The listing builds one solid part. Answer for the finished solid, in the listing's coordinates (mm). A direction names the side the tool comes from. Round coordinates to 2 decimals unless told otherwise and drop trailing zeros. Order: outer loops, then holes, each group sorted by start corner. A loop starts at its lowest first (then second) coordinate and runs counter-clockwise, first axis right, second up. Notation, with made-up numbers: (23.5, 75) - (67.5, 75) arc R19 cw to (67.5, 99) - close; hole circle Ø1 at (24.5, -30). An arc over 180 degrees is marked (long way). Write item = value, one per line.
from build123d import *

# Parameters (mm, degrees)
ESBO_O1_R                     = 35
ESBO_O1_R_2                   = 32.5
RESSALTO_EXTRUS_O1_DEPTH      = 8
RESSALTO_EXTRUS_O2_START      = -3
ESBO_O2_R                     = 32.5
RESSALTO_EXTRUS_O2_DEPTH      = 3
ESBO_O3_R                     = 2.5
CORTE_EXTRUS_O1_DEPTH         = 3
RESSALTO_EXTRUS_O3_DEPTH      = 5
RESSALTO_EXTRUS_O3_DEPTH_BACK = 3
ESBO_O4_R                     = 37
ESBO_O4_R_2                   = 35
ESBO_O5_W                     = 1.8
ESBO_O5_H                     = 3
ESBO_O6_R                     = 12.55
RESSALTO_EXTRUS_O4_DEPTH      = 5
CORTE_EXTRUS_O2_DEPTH         = 53.933921071
CORTE_EXTRUS_O2_DEPTH_BACK    = 53.933921071
ESBO_O7_R                     = 7.55
RESSALTO_EXTRUS_O5_START      = -8
ESBO_O8_R                     = 37
ESBO_O8_R_2                   = 32.5
RESSALTO_EXTRUS_O5_DEPTH      = 8
ESBO_O9_R                     = 37
ESBO_O9_R_2                   = 33.5
CORTE_EXTRUS_O8_DEPTH         = 1.5
CORTE_EXTRUS_O9_START         = -1.5
ESBO_O12_R                    = 37
ESBO_O12_R_2                  = 33.5
CORTE_EXTRUS_O9_DEPTH         = 1.5
CORTE_EXTRUS_O10_START        = -10
ESBO_O13_R                    = 37
ESBO_O13_R_2                  = 36
CORTE_EXTRUS_O10_DEPTH        = 10
ESBO_O14_R                    = 37
ESBO_O14_R_2                  = 36
RESSALTO_EXTRUS_O6_DEPTH      = 5
ESBO_O15_R                    = 12.55
CORTE_EXTRUS_O11_DEPTH        = 53.933921071
ESBO_O16_R                    = 12.55
RESSALTO_EXTRUS_O7_DEPTH      = 3
ESBO_O17_R                    = 10
RESSALTO_EXTRUS_O8_DEPTH      = 16
ESBO_O18_R                    = 2.5
CORTE_EXTRUS_O12_DEPTH        = 56.668662639
ESBO_O19_W                    = 5.95
ESBO_O19_H                    = 2.65
CORTE_EXTRUS_O13_DEPTH        = 8
CORTE_EXTRUS_O14_DEPTH        = 57.676714795
CORTE_EXTRUS_O14_DEPTH_BACK   = 57.676714795
ESBO_O21_R                    = 1.65
ESBO_O23_R                    = 37
ESBO_O23_R_2                  = 36
CORTE_EXTRUS_O15_DEPTH        = 54.798234195


with BuildPart() as part:
    # Esboço1 → Ressalto-extrusão1 (new body)
    with BuildSketch(Plane.XY):
        Circle(ESBO_O1_R)
        Circle(ESBO_O1_R_2, mode=Mode.SUBTRACT)
    extrude(amount=RESSALTO_EXTRUS_O1_DEPTH)

    # Esboço2 → Ressalto-extrusão2 (add)
    with BuildSketch(Plane.XY.offset(8).offset(RESSALTO_EXTRUS_O2_START)):
        Circle(ESBO_O2_R)
    extrude(amount=RESSALTO_EXTRUS_O2_DEPTH)

    # Esboço3 → Corte-extrusão1 (cut)
    with BuildSketch(Plane.XY.offset(8)):
        Circle(ESBO_O3_R)
    extrude(amount=-CORTE_EXTRUS_O1_DEPTH, mode=Mode.SUBTRACT)

    # Esboço4 → Ressalto-extrusão3 (add, two sides: drawn at the far end of the back side and taken through both)
    with BuildSketch(Plane(origin=(0, 0, 5), x_dir=(-1, 0, 0), z_dir=(0, 0, -1)).offset(-RESSALTO_EXTRUS_O3_DEPTH_BACK)):
        Circle(ESBO_O4_R)
        Circle(ESBO_O4_R_2, mode=Mode.SUBTRACT)
    extrude(amount=RESSALTO_EXTRUS_O3_DEPTH + RESSALTO_EXTRUS_O3_DEPTH_BACK)

    # Esboço5 → Corte-Revolução1 (revolve, cut)
    with BuildSketch(Plane(origin=(0, 0, 0), x_dir=(1, 0, 0), z_dir=(0, 1, 0))):
        with Locations((-36.1, -2.5)):
            Rectangle(ESBO_O5_W, ESBO_O5_H)
        with Locations((-36.1, -5.5)):
            Rectangle(ESBO_O5_W, ESBO_O5_H)
    revolve(axis=Axis((0, 0, 8), (0, 0, -1)), mode=Mode.SUBTRACT)

    # Esboço6 → Ressalto-extrusão4 (add)
    with BuildSketch(Plane(origin=(0, 0, 5), x_dir=(-1, 0, 0), z_dir=(0, 0, -1))):
        with Locations(Location((0, 0, 0), (0, 0, 180))):
            Circle(ESBO_O6_R)
    extrude(amount=RESSALTO_EXTRUS_O4_DEPTH)

    # Esboço7 → Corte-extrusão2 (cut, two sides: drawn at the far end of the back side and taken through both)
    with BuildSketch(Plane(origin=(0, 0, 0), x_dir=(-1, 0, 0), z_dir=(0, 0, -1)).offset(-CORTE_EXTRUS_O2_DEPTH_BACK)):
        Circle(ESBO_O7_R)
    extrude(amount=CORTE_EXTRUS_O2_DEPTH + CORTE_EXTRUS_O2_DEPTH_BACK, mode=Mode.SUBTRACT)

    # Esboço8 → Ressalto-extrusão5 (add)
    with BuildSketch(Plane.XY.offset(8).offset(RESSALTO_EXTRUS_O5_START)):
        with Locations(Location((0, 0, 0), (0, 0, 180))):
            Circle(ESBO_O8_R)
        Circle(ESBO_O8_R_2, mode=Mode.SUBTRACT)
    extrude(amount=RESSALTO_EXTRUS_O5_DEPTH)

    # Esboço9 → Corte-extrusão8 (cut)
    with BuildSketch(Plane.XY.offset(8)):
        with Locations(Location((0, 0, 0), (0, 0, 180))):
            Circle(ESBO_O9_R)
        Circle(ESBO_O9_R_2, mode=Mode.SUBTRACT)
    extrude(amount=-CORTE_EXTRUS_O8_DEPTH, mode=Mode.SUBTRACT)

    # Esboço12 → Corte-extrusão9 (cut)
    with BuildSketch(Plane(origin=(0, 0, 0), x_dir=(-1, 0, 0), z_dir=(0, 0, -1)).offset(CORTE_EXTRUS_O9_START)):
        Circle(ESBO_O12_R)
        with Locations(Location((0, 0, 0), (0, 0, 180))):
            Circle(ESBO_O12_R_2, mode=Mode.SUBTRACT)
    extrude(amount=CORTE_EXTRUS_O9_DEPTH, mode=Mode.SUBTRACT)

    # Esboço13 → Corte-extrusão10 (cut)
    with BuildSketch(Plane(origin=(0, 0, 1.5), x_dir=(-1, 0, 0), z_dir=(0, 0, -1)).offset(CORTE_EXTRUS_O10_START)):
        Circle(ESBO_O13_R)
        Circle(ESBO_O13_R_2, mode=Mode.SUBTRACT)
    extrude(amount=CORTE_EXTRUS_O10_DEPTH, mode=Mode.SUBTRACT)

    # Esboço14 → Ressalto-extrusão6 (add)
    with BuildSketch(Plane.XY.offset(6.5)):
        Circle(ESBO_O14_R)
        Circle(ESBO_O14_R_2, mode=Mode.SUBTRACT)
    extrude(amount=-RESSALTO_EXTRUS_O6_DEPTH)

    # Esboço15 → Corte-extrusão11 (cut, through all)
    with BuildSketch(Plane(origin=(0, 0, 0), x_dir=(-1, 0, 0), z_dir=(0, 0, -1))):
        Circle(ESBO_O15_R)
    extrude(amount=-CORTE_EXTRUS_O11_DEPTH, mode=Mode.SUBTRACT)

    # Esboço16 → Ressalto-extrusão7 (add, through all)
    with BuildSketch(Plane(origin=(0, 0, 5), x_dir=(-1, 0, 0), z_dir=(0, 0, -1))):
        Circle(ESBO_O16_R)
    extrude(amount=-RESSALTO_EXTRUS_O7_DEPTH)

    # Esboço17 → Ressalto-extrusão8 (add)
    with BuildSketch(Plane(origin=(0, 0, 5), x_dir=(-1, 0, 0), z_dir=(0, 0, -1))):
        with Locations(Location((0, 0, 0), (0, 0, 180))):
            Circle(ESBO_O17_R)
    extrude(amount=RESSALTO_EXTRUS_O8_DEPTH)

    # Esboço18 → Corte-extrusão12 (cut, through all)
    with BuildSketch(Plane(origin=(0, 0, -11), x_dir=(-1, 0, 0), z_dir=(0, 0, -1))):
        Circle(ESBO_O18_R)
    extrude(amount=-CORTE_EXTRUS_O12_DEPTH, mode=Mode.SUBTRACT)

    # Esboço19 → Corte-extrusão13 (cut)
    with BuildSketch(Plane(origin=(0, 0, -11), x_dir=(-1, 0, 0), z_dir=(0, 0, -1))):
        with Locations((0, -5.825)):
            Rectangle(ESBO_O19_W, ESBO_O19_H)
        with Locations((0, 5.825)):
            Rectangle(ESBO_O19_W, ESBO_O19_H)
    extrude(amount=-CORTE_EXTRUS_O13_DEPTH, mode=Mode.SUBTRACT)

    # Esboço21 → Corte-extrusão14 (cut, two sides: drawn at the far end of the back side and taken through both)
    with BuildSketch(Plane(origin=(0, 4.5, 0), x_dir=(1, 0, 0), z_dir=(0, 1, 0)).offset(-CORTE_EXTRUS_O14_DEPTH_BACK)):
        with Locations(Location((0, 6.85, 0), (0, 0, 180))):
            Circle(ESBO_O21_R)
    extrude(amount=CORTE_EXTRUS_O14_DEPTH + CORTE_EXTRUS_O14_DEPTH_BACK, mode=Mode.SUBTRACT)

    # Esboço23 → Corte-extrusão15 (cut, through all)
    with BuildSketch(Plane(origin=(0, 0, 1.5), x_dir=(-1, 0, 0), z_dir=(0, 0, -1))):
        Circle(ESBO_O23_R)
        Circle(ESBO_O23_R_2, mode=Mode.SUBTRACT)
    extrude(amount=-CORTE_EXTRUS_O15_DEPTH, mode=Mode.SUBTRACT)


solid = part.part
Q1. Section C-C on x = 0 is taken. Count the separate pieces of the cut face and the enclosed holes in it, then the cut area to 3 significant figures.
Model answer:
separate_pieces = 6
enclosed_holes = 0
area = 387 mm^2
Q2. Find the intervals of material crossed by line 1 (Y direction, x = 0, z = 4.5); line 2 (Z direction, x = 0, y = 8); line 3 (Y direction, x = 7.5, z = 1.25), in increasing order. Write a range as from..to.
Model answer:
line_1 = -36..-32.5, -10..-2.5, 2.5..10, 32.5..36
line_2 = -11..-8.5, -5.2..8
line_3 = -32.65..-31.62, -6.61..6.61, 31.62..32.65
Q3. Section A-A on y = 0 is taken. Determine the outline of the cut face in (x, z).
Model answer:
outline = (-36, 1.5) - (-33.5, 1.5) - (-33.5, 0) - (-32.5, 0) - (-32.5, 5) - (-10, 5) - (-10, -11) - (-2.5, -11) - (-2.5, 8) - (-33.5, 8) - (-33.5, 6.5) - (-36, 6.5) - close; (2.5, -11) - (10, -11) - (10, 5) - (32.5, 5) - (32.5, 0) - (33.5, 0) - (33.5, 1.5) - (36, 1.5) - (36, 6.5) - (33.5, 6.5) - (33.5, 8) - (2.5, 8) - close
Q4. Section D-D on y = -8 is taken. Determine the outline of the cut face in (x, z), then the cut area to 3 significant figures.
Model answer:
outline = (-35.1, 1.5) - (-32.53, 1.5) - (-32.53, 0) - (-31.5, 0) - (-31.5, 5) - (-6, 5) - (-6, -11) - (6, -11) - (6, 5) - (31.5, 5) - (31.5, 0) - (32.53, 0) - (32.53, 1.5) - (35.1, 1.5) - (35.1, 6.5) - (32.53, 6.5) - (32.53, 8) - (-32.53, 8) - (-32.53, 6.5) - (-35.1, 6.5) - close; hole circle Ø3.3 at (0, -6.85)
area = 415 mm^2
Q5. For faces 1 (the face through (0, 6, -3)), 2 (the face through (-1.574, -8.597, -6.354)), determine the directions among +Z, -Z, +X, -X, +Y, -Y from which every point of the face is accessible in a straight line to the end or side of a thin tool.
Model answer:
face_1 = -Z
face_2 = +Y, -Y
Q6. Flat-ended cylindrical pins translate along their axes: P1, Ø2, axis at y = 5.5, z = -5.5, coming from the +X side; P2, Ø8, axis at y = -9, z = 0.5, coming from the +X side; P3, Ø2, axis at y = 5.5, z = -6.5, coming from the -X side; P4, Ø2.5, axis at x = 0, z = -6.85, coming from the +Y side. Find the tip coordinate at first contact, or state that the pin passes through.
Model answer:
P1 = 8.93
P2 = 35.63
P3 = -8.93
P4 = through
Q7. Section B-B on z = -6.85 is taken. Determine the outline of the cut face in (x, y) (3 decimals), then the cut area to 3 significant figures.
Model answer:
outline = (-2.975, -7.15) - (-2.975, -4.5) - (-1.65, -4.5) - (-1.65, -1.878) arc R2.5 cw to (-1.65, 1.878) - (-1.65, 4.5) - (-2.975, 4.5) - (-2.975, 7.15) - (-1.65, 7.15) - (-1.65, 9.863) arc R10 ccw to (-1.65, -9.863) - (-1.65, -7.15) - close; (1.65, -9.863) arc R10 ccw to (1.65, 9.863) - (1.65, 7.15) - (2.975, 7.15) - (2.975, 4.5) - (1.65, 4.5) - (1.65, 1.878) arc R2.5 cw to (1.65, -1.878) - (1.65, -4.5) - (2.975, -4.5) - (2.975, -7.15) - (1.65, -7.15) - close
area = 230 mm^2
Q8. Determine the mould class of faces 3 (the face through (24, -24, 1.5)), 4 (the face through (-7.262, -32.703, 7.26)), 5 (the face through (-1.574, -3.499, -6.354)) for opening direction Z: released by +Z, released by -Z, zero draft, split by the parting line, or undercut.
Model answer:
face_3 = released by -Z
face_4 = zero draft
face_5 = undercut
